Autodesk Inventor part; units mm, degrees
ref_plane "YZ Plane" through (0, 0, 0) normal (1, 0, 0) x (0, 1, 0)
ref_plane "XZ Plane" through (0, 0, 0) normal (0, 1, 0) x (-1, 0, 0)
ref_plane "XY Plane" through (0, 0, 0) normal (0, 0, 1) x (1, 0, 0)
sketch "スケッチ1" plane through (0, 0, 0) normal (0, 1, 0) x (-1, 0, 0)
  line L0 (0, 0) -> (180, 0)
  line L1 (180, 0) -> (180, -90)
  line L2 (180, -90) -> (0, -90)
  line L3 (0, -90) -> (0, 0)
  line L4 (20, -10) -> (10, -10)
  line L5 (10, -10) -> (10, -14)
  line L6 (10, -14) -> (20, -14)
  line L7 (20, -14) -> (20, -10)
  line L8 (20, -76) -> (10, -76)
  line L9 (10, -76) -> (10, -80)
  line L10 (10, -80) -> (20, -80)
  line L11 (20, -80) -> (20, -76)
  line L12 (40, -76) -> (30, -76)
  line L13 (30, -76) -> (30, -80)
  line L14 (30, -80) -> (40, -80)
  line L15 (40, -80) -> (40, -76)
  line L16 (40, -10) -> (30, -10)
  line L17 (30, -10) -> (30, -14)
  line L18 (40, -14) -> (40, -10)
  line L19 (30, -14) -> (40, -14)
  line L20 (60, -76) -> (50, -76)
  line L21 (50, -76) -> (50, -80)
  line L22 (50, -80) -> (60, -80)
  line L23 (60, -80) -> (60, -76)
  line L24 (60, -10) -> (50, -10)
  line L25 (50, -10) -> (50, -14)
  line L26 (60, -14) -> (60, -10)
  line L27 (50, -14) -> (60, -14)
  line L28 (80, -76) -> (70, -76)
  line L29 (70, -76) -> (70, -80)
  line L30 (70, -80) -> (80, -80)
  line L31 (80, -80) -> (80, -76)
  line L32 (80, -10) -> (70, -10)
  line L33 (70, -10) -> (70, -14)
  line L34 (80, -14) -> (80, -10)
  line L35 (70, -14) -> (80, -14)
  line L36 (100, -76) -> (90, -76)
  line L37 (90, -76) -> (90, -80)
  line L38 (90, -80) -> (100, -80)
  line L39 (100, -80) -> (100, -76)
  line L40 (100, -10) -> (90, -10)
  line L41 (90, -10) -> (90, -14)
  line L42 (100, -14) -> (100, -10)
  line L43 (90, -14) -> (100, -14)
  line L44 (120, -76) -> (110, -76)
  line L45 (110, -76) -> (110, -80)
  line L46 (110, -80) -> (120, -80)
  line L47 (120, -80) -> (120, -76)
  line L48 (120, -10) -> (110, -10)
  line L49 (110, -10) -> (110, -14)
  line L50 (120, -14) -> (120, -10)
  line L51 (110, -14) -> (120, -14)
  line L52 (140, -76) -> (130, -76)
  line L53 (130, -76) -> (130, -80)
  line L54 (130, -80) -> (140, -80)
  line L55 (140, -80) -> (140, -76)
  line L56 (140, -10) -> (130, -10)
  line L57 (130, -10) -> (130, -14)
  line L58 (140, -14) -> (140, -10)
  line L59 (130, -14) -> (140, -14)
  line L60 (160, -76) -> (150, -76)
  line L61 (150, -76) -> (150, -80)
  line L62 (150, -80) -> (160, -80)
  line L63 (160, -80) -> (160, -76)
  line L64 (160, -10) -> (150, -10)
  line L65 (150, -10) -> (150, -14)
  line L66 (160, -14) -> (160, -10)
  line L67 (150, -14) -> (160, -14)
  line L68 (180, -20) -> (176, -20)
  line L69 (176, -20) -> (176, -30)
  line L70 (176, -30) -> (180, -30)
  line L71 (180, -30) -> (180, -20)
  line L72 (176, -40) -> (176, -50)
  line L73 (180, -40) -> (176, -40)
  line L74 (176, -50) -> (180, -50)
  line L75 (180, -50) -> (180, -40)
  line L76 (176, -60) -> (176, -70)
  line L77 (180, -60) -> (176, -60)
  line L78 (176, -70) -> (180, -70)
  line L79 (180, -70) -> (180, -60)
  circle A0 centre (5, -5) radius 1.55
  circle A1 centre (5, -85) radius 1.55
  circle A2 centre (175, -85) radius 1.55
  circle A3 centre (175, -5) radius 1.55
  point P0 (10, -78)
  point P1 (30, -78)
  point P2 (50, -78)
  point P3 (70, -78)
  point P4 (90, -78)
  point P5 (110, -78)
  point P6 (130, -78)
  point P7 (150, -78)
  dimension "d0" = 180
  dimension "d1" = 90
  dimension "d2" = 10
  dimension "d3" = 4
  dimension "d4" = 10
  dimension "d5" = 10
  dimension "d6" = 10
  dimension "d7" = 4
  dimension "d8" = 10
  dimension "d9" = 10
  dimension "d12" = 20
  dimension "d17" = 4
  dimension "d18" = 10
  dimension "d19" = 20
  dimension "d22" = 20
  dimension "d27" = 0
  dimension "d28" = 3.1
  dimension "d29" = 3.1
  dimension "d30" = 3.1
  dimension "d31" = 3.1
  dimension "d32" = 5
  dimension "d33" = 5
  dimension "d34" = 5
  dimension "d35" = 5
  dimension "d36" = 5
  dimension "d37" = 5
  dimension "d39" = 5
  dimension "d40" = 5
extrude "押し出し1" add sketch "スケッチ1" along normal blind 4 contours L0 L1 L68 L69 L70 L73 L72 L74 L77 L76 L78 L2 L3
properties part number "ER_lipo_bottom_1" material "木材 (オーク)"
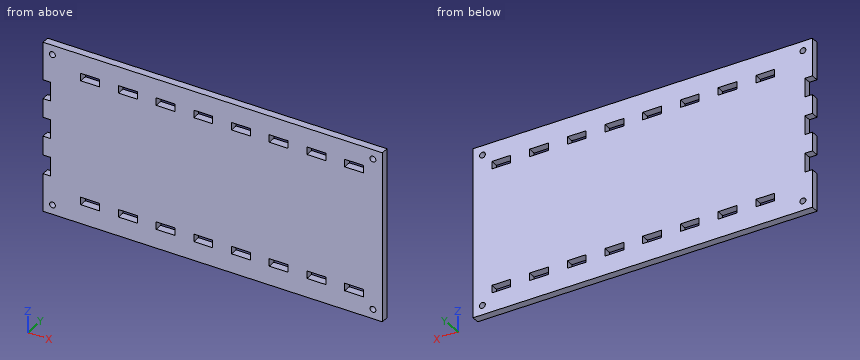
Build history of the part. All positions in model axes, mm. Coordinates: 2 decimals unless noted, no trailing zeros. Write each loop counter-clockwise with the first axis right and the second up, starting at its lowest first coordinate (ties: lowest second). Pieces come first, ordered by that corner, then holes.
1. Band-saw the part on B-B, the plane y = 2. Give the number of separate pieces and of enclosed holes in the cut face, and give its area (3 significant figures).
Answer block:
separate pieces: 1
enclosed holes: 20
area: 15,400 mm2
2. Band-saw the part on A-A, the plane x = -14. Give the cut face in (y, z).
Answer block:
outline: (0, -90) - (4, -90) - (4, -80) - (0, -80) - close; (0, -76) - (4, -76) - (4, -14) - (0, -14) - close; (0, -10) - (4, -10) - (4, 0) - (0, 0) - close
3. Drill centre lines: probe 1 along Z at (x, y) = (-130.5, 0.3); probe 2 along Z at (x, y) = (-5, 2.15); probe 3 along X at (y, z) = (1.75, -85). Where is each one in solid material? Low to high.
Answer block:
probe 1: z = -90 to -80, -76 to -14, -10 to 0
probe 2: z = -90 to -86.55, -83.45 to -6.55, -3.45 to 0
probe 3: x = -180 to -176.55, -173.45 to -6.55, -3.45 to 0
